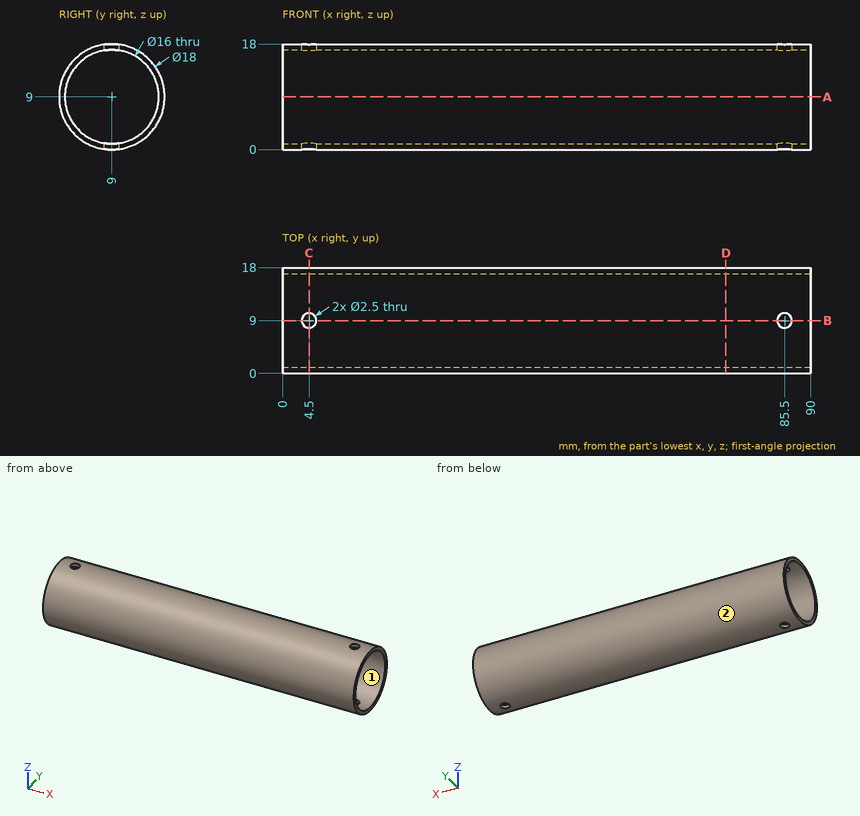
Source: three-view drawing plus pictorial views. Frame: mm from the lowest corner of the part. Coordinates: 2 decimals unless noted, no trailing zeros. Loops run counter-clockwise (first coordinate to the right, second up) from the corner with the lowest first, then second, coordinate; pieces in that order, holes last. Notation, with made-up numbers: (22, 89) - (58, 89) arc R17 cw to (58, 116) - close; hole circle Ø5 at (16, 60.25). An arc over 180 degrees is marked (long way). Answer in a Markdown table with one row per item. Add a question column.
Item 1: Section query A-A on z = 9. Return the cut outline in (x, y), then the cut area to 3 significant figures.
Item 2: Section query D-D on x = 75.5. Return the cut outline in (y, z), then the cut area to 3 significant figures.
Item 3: Mould query, pull axis Z, two halves, no side actions, for the marked faces 1 and 2. Classes: released by +Z, released by -Z, zero draft, split by the parting line, or undercut.
Item 4: Contact query for flat-ended pins moving along their axis: P1, Ø10, axis at x = 40, y = 14.5, coming from the +Z side; P2, Ø4, axis at x = 62, y = 5.5, coming from the -Z side; P3, Ø10, axis at x = 40, z = 14.5, coming from the -Y side. Output: stop coordinate, or through.
Item 5: Line query: line 1 along Z through (x, y) = (68, 8.75); line 2 along Z through (x, y) = (56.5, 11); line 3 along Y through (x, z) = (77, 7.5). Output: solid intervals per line, ascending. Write a range as [from, to].
Item 6: Section query C-C on x = 4.5. Return the cut outline in (y, z).
Item 7: Section query B-B on y = 9. Return the cut outline in (x, z).
Recorded:
| question | item | result |
|---|---|---|
| 1 | outline | (0, 0) - (90, 0) - (90, 1) - (0, 1) - close; (0, 17) - (90, 17) - (90, 18) - (0, 18) - close |
| 1 | area | 180 mm^2 |
| 2 | outline | circle Ø18 at (9, 9); hole circle Ø16 at (9, 9) |
| 2 | area | 53.4 mm^2 |
| 3 | face 1 | undercut |
| 3 | face 2 | split by the parting line |
| 4 | P1 | z = 17.99 |
| 4 | P2 | z = 0.13 |
| 4 | P3 | y = 0.01 |
| 5 | line 1 | [0, 1], [17, 18] |
| 5 | line 2 | [0.23, 1.25], [16.75, 17.77] |
| 5 | line 3 | [0.13, 1.14], [16.86, 17.87] |
| 6 | outline | (7.75, 0.09) - (7.75, 1.1) arc R8 cw to (7.75, 16.9) - (7.75, 17.91) arc R9 ccw to start; (10.25, 0.09) arc R9 ccw to (10.25, 17.91) - (10.25, 16.9) arc R8 cw to (10.25, 1.1) - close |
| 7 | outline | (0, 0) - (3.25, 0) - (3.25, 1) - (0, 1) - close; (0, 17) - (3.25, 17) - (3.25, 18) - (0, 18) - close; (5.75, 0) - (84.25, 0) - (84.25, 1) - (5.75, 1) - close; (5.75, 17) - (84.25, 17) - (84.25, 18) - (5.75, 18) - close; (86.75, 0) - (90, 0) - (90, 1) - (86.75, 1) - close; (86.75, 17) - (90, 17) - (90, 18) - (86.75, 18) - close |
